Here's how the part is built. I have some questions about the finished solid (model axes, mm). A direction names the side the tool comes from. Round coordinates to 2 decimals unless told otherwise and drop trailing zeros. Order: outer loops, then holes, each group sorted by start corner. A loop starts at its lowest first (then second) coordinate and runs counter-clockwise, first axis right, second up. Notation, with made-up numbers: (-28, 69.25) -> (21, 69.25) arc R17 cw to (21, 74.25) -> close; hole circle Ø4 at (54, 52). An arc over 180 degrees is marked (long way). Answer in a Markdown table with one row per item.
```python
from build123d import *

# Parameters (mm, degrees)
BASE_FLANGE1_START                     = -44.45
BASE_FLANGE1_DEPTH                     = 44.45
SKETCH2_R                              = 3.175
CE_00_HOLES_0_250_SIDE_2_PLACES_DEPTH  = 7.62
SKETCH4_R                              = 3.175
CE_00_HOLES_0_250_ANGLED_1_PLACE_DEPTH = 7.62


# Read off the part's stored shape, not the designer's step: Base-Flange1
with BuildPart() as part:
    # Base-Flange1 outline → Base-Flange1 (new body)
    with BuildSketch(Plane.XY.offset(BASE_FLANGE1_START)):
        with BuildLine():
            ThreePointArc((0.146646968, 139.954), (-0.039293937, 139.768059095), (-0.293293937, 139.7))
            Line((-0.293293937, 139.7), (-6.35, 139.7))
            Line((-6.35, 139.7), (-6.35, 137.414))
            Line((-6.35, 137.414), (-0.293293937, 137.414))
            ThreePointArc((-0.293293937, 137.414), (1.103706063, 137.788325022), (2.126381041, 138.811))
            Line((2.126381041, 138.811), (2.492998462, 139.446))
            ThreePointArc((2.492998462, 139.446), (2.678939367, 139.631940905), (2.932939367, 139.7))
            Line((2.932939367, 139.7), (62.784570335, 139.7))
            ThreePointArc((62.784570335, 139.7), (63.44554116, 139.568524729), (64.005885168, 139.194114832))
            Line((64.005885168, 139.194114832), (139.194114832, 64.005885168))
            ThreePointArc((139.194114832, 64.005885168), (139.568524729, 63.44554116), (139.7, 62.784570335))
            Line((139.7, 62.784570335), (139.7, -200.267060633))
            ThreePointArc((139.7, -200.267060633), (139.631940905, -200.521060633), (139.446, -200.707001538))
            Line((139.446, -200.707001538), (138.811, -201.073618959))
            ThreePointArc((138.811, -201.073618959), (137.788325022, -202.096293937), (137.414, -203.493293937))
            Line((137.414, -203.493293937), (137.414, -209.55))
            Line((137.414, -209.55), (139.7, -209.55))
            Line((139.7, -209.55), (139.7, -203.493293937))
            ThreePointArc((139.7, -203.493293937), (139.768059095, -203.239293937), (139.954, -203.053353032))
            Line((139.954, -203.053353032), (140.589, -202.686735611))
            ThreePointArc((140.589, -202.686735611), (141.611674978, -201.664060633), (141.986, -200.267060633))
            Line((141.986, -200.267060633), (141.986, 62.784570335))
            ThreePointArc((141.986, 62.784570335), (141.68051334, 64.320355486), (140.810560934, 65.622331269))
            Line((140.810560934, 65.622331269), (65.622331269, 140.810560934))
            ThreePointArc((65.622331269, 140.810560934), (64.320355486, 141.68051334), (62.784570335, 141.986))
            Line((62.784570335, 141.986), (2.932939367, 141.986))
            ThreePointArc((2.932939367, 141.986), (1.535939367, 141.611674978), (0.513264389, 140.589))
            Line((0.513264389, 140.589), (0.146646968, 139.954))
        make_face()
    extrude(amount=BASE_FLANGE1_DEPTH)

    # Sketch2 → CE-00 Holes 0.250 Side 2 Places (cut)
    with BuildSketch(Plane(origin=(141.986, 0, 0), x_dir=(0, 0, -1), z_dir=(1, 0, 0))):
        with Locations(Location((22.225, 11.1252, 0), (0, 0, 90))):
            Circle(SKETCH2_R)
        with Locations(Location((22.225, -103.1748, 0), (0, 0, 90))):
            Circle(SKETCH2_R)
    extrude(amount=-CE_00_HOLES_0_250_SIDE_2_PLACES_DEPTH, mode=Mode.SUBTRACT)

    # Sketch4 → CE-00 Holes 0.250 Angled 1 Place (cut)
    with BuildSketch(Plane(origin=(103.216446102, 103.216446102, 0), x_dir=(0, 0, -1), z_dir=(0.7071067811865511, 0.7071067811865439, 0))):
        with Locations(Location((22.225, 2.366107061, 0), (0, 0, 90))):
            Circle(SKETCH4_R)
    extrude(amount=-CE_00_HOLES_0_250_ANGLED_1_PLACE_DEPTH, mode=Mode.SUBTRACT)


solid = part.part
```
1. For pin 1 Ø13.5 at (x, z) = (44, -22) entering from -Y; pin 2 Ø4 at (y, z) = (-103.17, -22.22) entering from +X; pin 3 Ø12 at (x, z) = (90, -25) entering from +Y; pin 4 Ø13.5 at (y, z) = (-98, -24.5) entering from -X, each with a flat end and sliding along its axis, tell me the tip position at first contact or that it passes through.
Numbers:
| item | result |
|---|---|
| pin 1 | stops at y = 139.7 |
| pin 2 | passes through |
| pin 3 | stops at y = 122.43 |
| pin 4 | stops at x = 139.7 |
2. Please list where these lines run through material, in increasing order: line 1 along Y through (x, z) = (3.5, -21); line 2 along Y through (x, z) = (121, -38.5).
Numbers:
| item | result |
|---|---|
| line 1 | y = 139.7 to 141.99 |
| line 2 | y = 82.2 to 85.43 |
3. Suppose I cut it at A-A on z = -34. Write out the boundary of the cut face in (x, y).
Numbers:
| item | result |
|---|---|
| outline | (-6.35, 137.41) -> (-0.29, 137.41) arc R2.79 ccw to (2.13, 138.81) -> (2.49, 139.45) arc R0.51 cw to (2.93, 139.7) -> (62.78, 139.7) arc R1.73 cw to (64.01, 139.19) -> (139.19, 64.01) arc R1.73 cw to (139.7, 62.78) -> (139.7, -200.27) arc R0.51 cw to (139.45, -200.71) -> (138.81, -201.07) arc R2.79 ccw to (137.41, -203.49) -> (137.41, -209.55) -> (139.7, -209.55) -> (139.7, -203.49) arc R0.51 cw to (139.95, -203.05) -> (140.59, -202.69) arc R2.79 ccw to (141.99, -200.27) -> (141.99, 62.78) arc R4.01 ccw to (140.81, 65.62) -> (65.62, 140.81) arc R4.01 ccw to (62.78, 141.99) -> (2.93, 141.99) arc R2.79 ccw to (0.51, 140.59) -> (0.15, 139.95) arc R0.51 cw to (-0.29, 139.7) -> (-6.35, 139.7) -> close |
4. We'd pull the mould along Y, two halves only. Please class faces 1 (the face through (103.743, 102.69, -27.475)), 2 (the face through (140.859, 10.712, -19.077)), 3 (the face through (-3, 137.414, -23)): released by +Y, released by -Y, zero draft, split by the parting line, or undercut.
Numbers:
| item | result |
|---|---|
| face 1 | released by +Y |
| face 2 | undercut |
| face 3 | released by -Y |
5. For faces 4 (the face through (139.7, -67, -23)), 5 (the face through (32, 139.7, -23)), 6 (the face through (-3, 139.7, -23)), 7 (the face through (137.414, -206, -23)), 8 (the face through (139.7, -207, -23)), which set-ups out of +Z, -Z, +X, -X, +Y, -Y let a thin tool reach every point of the face, with its end or its side?
Numbers:
| item | result |
|---|---|
| face 4 | +Z, -Z, -X |
| face 5 | +Z, -Z, -Y |
| face 6 | +Z, -Z, -X, +Y |
| face 7 | +Z, -Z, -X, -Y |
| face 8 | +Z, -Z, +X, -Y |
6. Suppose I cut it at B-B on x = 36. Write out the boundary of the cut face in (y, z).
Numbers:
| item | result |
|---|---|
| outline | (139.7, -44.45) -> (141.99, -44.45) -> (141.99, 0) -> (139.7, 0) -> close |
